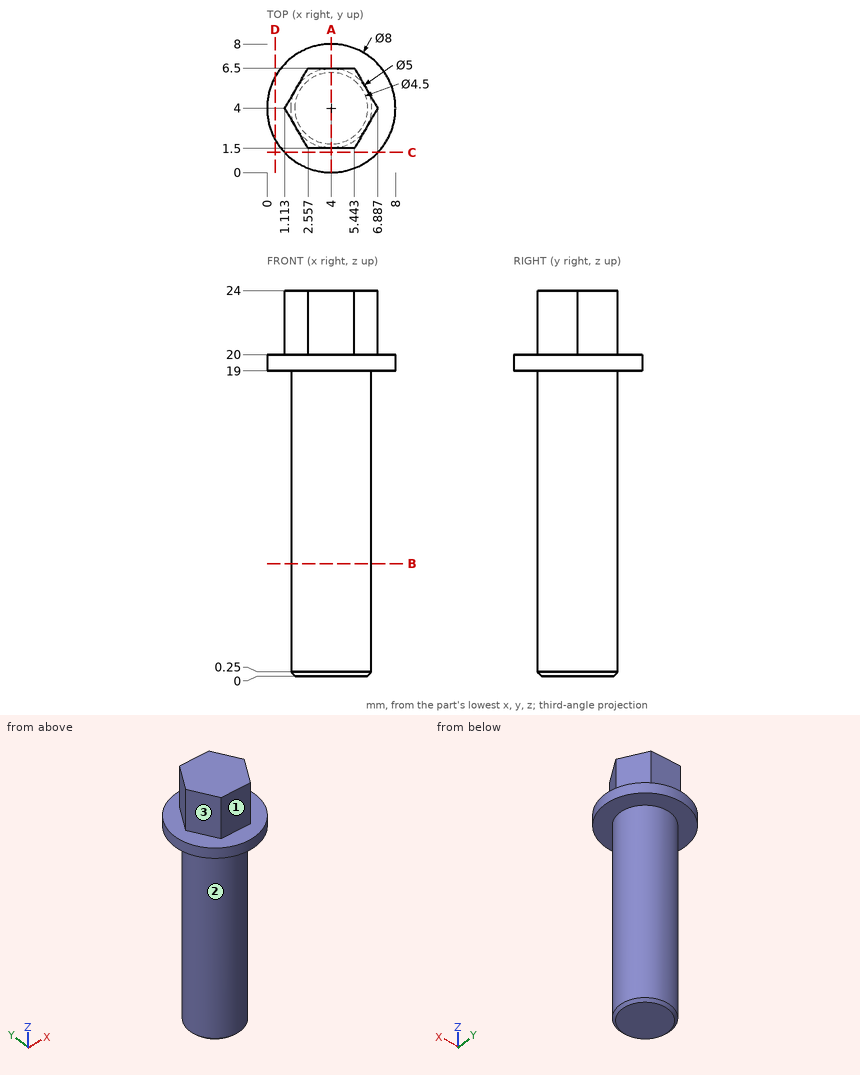
Part print with two shaded views. Sizes in mm from the minimum x, y, z corner. A direction names the side the tool comes from. Coordinates: 2 decimals unless noted, no trailing zeros. Write each loop counter-clockwise with the first axis right and the second up, starting at its lowest first coordinate (ties: lowest second). Pieces come first, ordered by that corner, then holes.
1. Band-saw the part on D-D, the plane x = 0.5. Give the cut face in (y, z).
Answer block:
outline: (2.06, 19) - (5.94, 19) - (5.94, 20) - (2.06, 20) - close
2. Band-saw the part on A-A, the plane x = 4. Give the cut face in (y, z).
Answer block:
outline: (0, 19) - (1.5, 19) - (1.5, 0.25) - (1.75, 0) - (6.25, 0) - (6.5, 0.25) - (6.5, 19) - (8, 19) - (8, 20) - (6.5, 20) - (6.5, 24) - (1.5, 24) - (1.5, 20) - (0, 20) - close
3. Band-saw the part on C-C, the plane y = 1.25. Give the cut face in (x, z) (1 decimal).
Answer block:
outline: (1.1, 19) - (6.9, 19) - (6.9, 20) - (1.1, 20) - close
4. Drop flat-ended pins along their axis: pin 1 (0.9 mm diameter, centred on x = 4, z = 21.5, fed in from -Y); pin 2 (1 mm diameter, centred on x = 1, y = 7, fed in from +Z); pin 3 (0.9 mm diameter, centred on x = 4.5, z = 21.5, fed in from +Y). Give the stop position or say it passes through.
Answer block:
pin 1: stops at y = 1.5
pin 2: stops at z = 20
pin 3: stops at y = 6.5
5. 3-axis set-ups, long thin cutter, end or side, ignore diameter. For the marked faces 1, 2 and 3: which of +Z, -Z, +X, -X, +Y, -Y reach the whole face in a straight line?
Answer block:
face 1: +Z, +X, -X, -Y
face 2: -Z
face 3: +Z, -X, -Y
6. Drill centre lines: probe 1 along Y at (x, z) = (2.75, 20.5); probe 2 along Z at (x, y) = (0.5, 3); probe 3 along Y at (x, z) = (5.75, 1.25) (1 decimal). Where is each one in solid material? Low to high.
Answer block:
probe 1: y = 1.5 to 6.5
probe 2: z = 19 to 20
probe 3: y = 2.2 to 5.8
7. Band-saw the part on B-B, the plane z = 7. Give the cut face in (x, y).
Answer block:
outline: circle Ø5 at (4, 4)
